from build123d import *

# Parameters (mm, degrees)
BOSS_EXTRUDE1_DEPTH  = 5
BOSS_EXTRUDE2_DEPTH  = 2.5
M4_CLEARANCE_HOLE2_D = 4.8
FILLET1_R            = 10
FILLET2_R            = 2.5


with BuildPart() as part:
    # Sketch1 → Boss-Extrude1 (new body)
    with BuildSketch(Plane(origin=(0, 0, 0), x_dir=(1, 0, 0), z_dir=(0, 1, 0))):
        Polygon((10.969655115, 19), (21.939310229, 0), (10.969655115, -19), (0, -19), (-10, -19), (-10, -16.5), (6.639528096, -16.5), (6.639528096, 16.5), (-10, 16.5), (-10, 19), (0, 19), align=None)
    extrude(amount=BOSS_EXTRUDE1_DEPTH)

    # Sketch2 → Boss-Extrude2 (add)
    with BuildSketch(Plane.XY.offset(19)):
        with BuildLine():
            Line((-10, 5), (-2, 5))
            ThreePointArc((-2, 5), (-6, 9), (-10, 5))
        make_face()
    boss_extrude2 = extrude(amount=-BOSS_EXTRUDE2_DEPTH)

    # Mirror1: Boss-Extrude2 across plane
    add(boss_extrude2.mirror(Plane.XY))

    # M4 Clearance Hole2 (through all)
    with Locations(Plane(origin=(-6, 5, 19), x_dir=(1, 0, 0), z_dir=(0, 0, 1))):
        with Locations((0, 0)):
            Hole(M4_CLEARANCE_HOLE2_D / 2)

    # Fillet1
    fillet1_edges = [part.edges().sort_by_distance(p)[0] for p in [
        (-2, 5, 17.75),
    ]]
    fillet(fillet1_edges, radius=FILLET1_R)

    # Fillet2
    fillet2_edges = [part.edges().sort_by_distance(p)[0] for p in [
        (-10, 0, 17.75),
        (-10, 0, -17.75),
        (10.969655115, 2.5, -19),
        (21.939310229, 2.5, 0),
        (10.969655115, 2.5, 19),
    ]]
    fillet(fillet2_edges, radius=FILLET2_R)


solid = part.part
Geometry: final body of the model. Coordinates: model frame, mm. A direction names the side the tool comes from. Give positions to 0.01 mm unless a question says otherwise; leave off trailing zeros. Write each loop counter-clockwise with the first axis right and the second up, starting at its lowest first coordinate (ties: lowest second). Pieces come first, ordered by that corner, then holes. Notation, with made-up numbers: M -6.5,-24.75 L 9.5,-24.75 A18 cw 9.5,-10.75 Z; hole C 9,76 d9. An arc over 180 degrees is marked long. Answer in a Markdown table with one row per item. Add a question column.
(1) Reachability of faces 4 (the flat face through (16.388, 2.465, -9.615)), 5 (the flat face through (-2, 4, -16.5)) from +Z, -Z, +X, -X, +Y, -Y: full face, straight path, thin tool, end or side. Return the list, or none.
(2) Section C-C on x = 1. Return loops of the section in (y, z).
(3) Section A-A on x = -6. Return loops of the section in (y, z), and give its area (3 significant figures).
(4) Section B-B on y = 3.75. Return loops of the section in (x, z), and give its area (3 significant figures).
(5) Mould query, pull axis Z, two halves, no side actions, for faces 1 (the cylindrical face through (10.792, 2.535, -18.656)), 2 (the cylindrical face through (-9.287, 0.752, 17.732)), 3 (the flat face through (6.64, 2, 0)). Classes: +Z half, -Z half, draft (parallel to the pull), parting line (faces both ways), or undercut.
(6) Ray query, line 1 (Y direction, x = -6, z = 17.3); line 2 (Z direction, x = -4, y = 3.5); line 3 (X direction, y = 1.75, z = 0). Return the intervals inside material, ascending.
(7) Section D-D on y = 6.5. Return loops of the section in (x, z).
(8) First-contact query: pin 1 (7 mm diameter, centred on x = 14, z = 0, fed in from +Y); pin 2 (2.5 mm diameter, centred on y = 3.5, z = -8, fed in from -X); pin 3 (3 mm diameter, centred on y = 1.5, z = 11.5, fed in from +X). Flat tips, straight axial feed; report the tip coordinate or a pass-through.
Result set:
| question | item | result |
|---|---|---|
| 1 | face 4 | -Z, +X, +Y, -Y |
| 1 | face 5 | -X, +Y, -Y |
| 2 | outline | M 0,-19 L 5,-19 L 5,-16.5 L 0,-16.5 Z; M 0,16.5 L 5.4,16.5 L 5.4,19 L 0,19 Z |
| 3 | outline | M 0,-19 L 2.6,-19 L 2.6,-16.5 L 0,-16.5 Z; M 0,16.5 L 2.6,16.5 L 2.6,19 L 0,19 Z; M 7.4,-19 L 9,-19 L 9,-16.5 L 7.4,-16.5 Z; M 7.4,16.5 L 9,16.5 L 9,19 L 7.4,19 Z |
| 3 | area | 21.0 mm^2 |
| 4 | outline | M -10,-19 L -8.05,-19 L -8.05,-16.5 L -10,-16.5 Z; M -10,16.5 L -8.05,16.5 L -8.05,19 L -10,19 Z; M -3.95,-19 L 9.53,-19 A2.5 ccw 11.69,-17.75 L 21.22,-1.25 A2.5 ccw 21.22,1.25 L 11.69,17.75 A2.5 ccw 9.53,19 L -3.95,19 L -3.95,16.5 L 6.64,16.5 L 6.64,-16.5 L -3.95,-16.5 Z |
| 4 | area | 435 mm^2 |
| 5 | face 1 | -Z half |
| 5 | face 2 | draft |
| 5 | face 3 | undercut |
| 6 | line 1 | y = 0 to 2.6, 7.4 to 9 |
| 6 | line 2 | z = -19 to -16.5, 16.5 to 19 |
| 6 | line 3 | x = 6.64 to 21.55 |
| 7 | outline | M -9.71,-19 L -7.87,-19 L -7.87,-16.5 L -9.71,-16.5 Z; M -9.71,16.5 L -7.87,16.5 L -7.87,19 L -9.71,19 Z; M -4.13,-19 L -2.29,-19 L -2.29,-16.5 L -4.13,-16.5 Z; M -4.13,16.5 L -1.47,16.5 L -1.47,19 L -4.13,19 Z |
| 8 | pin 1 | stops at y = 5 |
| 8 | pin 2 | stops at x = 6.64 |
| 8 | pin 3 | stops at x = 16.17 |
